from build123d import *

# Parameters (mm, degrees)
SKETCH1_W            = 20
SKETCH1_H            = 6
BOSS_EXTRUDE1_DEPTH  = 21.5
SKETCH2_W            = 6
SKETCH2_H            = 20
BOSS_EXTRUDE2_DEPTH  = 12
SKETCH7_R            = 1.5
CUT_EXTRUDE1_DEPTH   = 46.749316935
SKETCH8_R            = 3.4
CUT_EXTRUDE2_DEPTH   = 30.769951293
FILLET2_R            = 3
CONVERT_SOLID2_START = -10
CONVERT_SOLID2_DEPTH = 20


# Read off the part's stored shape, not the designer's step: Convert-Solid2
with BuildPart() as part:
    # Sketch1 → Boss-Extrude1 (new, symmetric)
    with BuildSketch(Plane(origin=(0, 0, 0), x_dir=(0, 0, -1), z_dir=(1, 0, 0))):
        with Locations((0, -3)):
            Rectangle(SKETCH1_W, SKETCH1_H)
    extrude(amount=BOSS_EXTRUDE1_DEPTH, both=True)

    # Sketch2 → Boss-Extrude2 (add)
    with BuildSketch(Plane(origin=(0, 0, 0), x_dir=(1, 0, 0), z_dir=(0, 1, 0))):
        with Locations((18.5, 0)):
            Rectangle(SKETCH2_W, SKETCH2_H)
        with Locations((-18.5, 0)):
            Rectangle(SKETCH2_W, SKETCH2_H)
    extrude(amount=BOSS_EXTRUDE2_DEPTH)

    # Sketch7 → Cut-Extrude1 (cut, through all)
    with BuildSketch(Plane.ZY.offset(21.5)):
        with Locations((-5, 7)):
            Circle(SKETCH7_R)
        with Locations((5, 7)):
            Circle(SKETCH7_R)
    extrude(amount=-CUT_EXTRUDE1_DEPTH, mode=Mode.SUBTRACT)

    # Sketch8 → Cut-Extrude2 (cut, through all)
    with BuildSketch(Plane.XZ.offset(6)):
        with Locations(Location((0, 0, 0), (0, 0, 270))):
            Circle(SKETCH8_R)
    extrude(amount=-CUT_EXTRUDE2_DEPTH, mode=Mode.SUBTRACT)

    # Fillet2
    fillet2_edges = [part.edges().sort_by_distance(p)[0] for p in [
        (-18.5, 12, 10),
        (-18.5, 12, -10),
        (18.5, 12, -10),
        (18.5, 12, 10),
    ]]
    fillet(fillet2_edges, radius=FILLET2_R)

    # Convert-Solid2 outline → Convert-Solid2 (cut)
    with BuildSketch(Plane.XY.offset(CONVERT_SOLID2_START)):
        with BuildLine():
            Line((21.5, -6), (21.5, 0))
            ThreePointArc((21.5, 0), (19.742640687, -4.242640687), (15.5, -6))
            Line((15.5, -6), (21.5, -6))
        make_face()
        with BuildLine():
            Line((-21.5, -6), (-15.5, -6))
            ThreePointArc((-15.5, -6), (-19.742640687, -4.242640687), (-21.5, 0))
            Line((-21.5, 0), (-21.5, -6))
        make_face()
        with BuildLine():
            Line((19.5, 0), (19.5, 12))
            Line((19.5, 12), (15.5, 12))
            Line((15.5, 12), (15.5, 0))
            Line((15.5, 0), (-15.5, 0))
            Line((-15.5, 0), (-15.5, 12))
            Line((-15.5, 12), (-19.5, 12))
            Line((-19.5, 12), (-19.5, 0))
            ThreePointArc((-19.5, 0), (-18.328427125, -2.828427125), (-15.5, -4))
            Line((-15.5, -4), (15.5, -4))
            ThreePointArc((15.5, -4), (18.328427125, -2.828427125), (19.5, 0))
        make_face()
    extrude(amount=CONVERT_SOLID2_DEPTH, mode=Mode.SUBTRACT)


solid = part.part
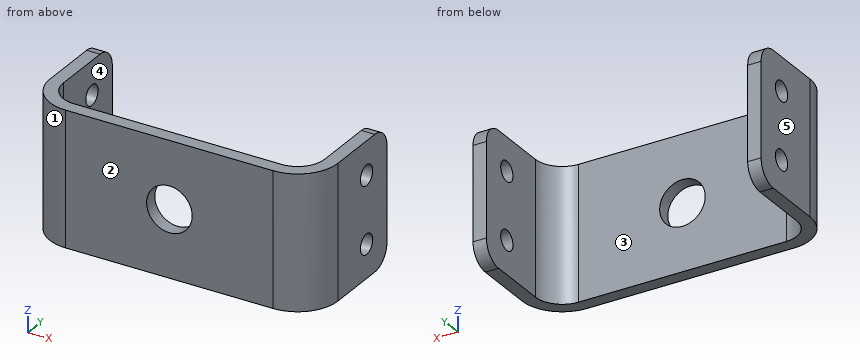
Check sheet for the modelled part. Datum: model origin and axes. Units: mm. Face numbers are marked on the shaded views. A direction names the side the tool comes from. Coordinates: 2 decimals unless noted, no trailing zeros. Loops run counter-clockwise (first coordinate to the right, second up) from the corner with the lowest first, then second, coordinate; pieces in that order, holes last. Notation, with made-up numbers: (42, 82) -> (80, 82) arc R13 cw to (80, 98) -> close; hole circle Ø11 at (-38.75, 70.5). An arc over 180 degrees is marked (long way). Write item = value, one per line. Start each with the question number.
1. Section check C-C on z = 0. Record the cut outline in (x, y).
2. Draft check along X on the marked faces 1, 2 and 3. Enter one of: released by +X, released by -X, zero draft, split by the parting line, or undercut.
3. Section check B-B on z = -5. Record the cut outline in (x, y), then the cut area to 3 significant figures.
4. Depth check by flat-ended pin: P1, Ø10, axis at y = -1, z = -4, coming from the +X side. Enter the tip coordinate at first touch or a pass-through.
5. Tool access check on the marked faces 4 and 5. Record the directions out of +Z, -Z, +X, -X, +Y, -Y that give a thin tool (end or side, any length) a straight path to the whole face; none if there is none.
6. Section check A-A on y = 7. Record the cut outline in (x, z).
7. Material ranges on line 1 (X direction, y = 7, z = -2); line 2 (Y direction, x = 13, z = 1.75); line 3 (X direction, y = -4.6, z = 0), recorded low to high.
8. Section check D-D on y = 4.5. Record the cut outline in (x, z), then the cut area to 3 significant figures.
Responses:
q1.outline = (-21.5, 0) arc R6 ccw to (-15.5, -6) -> (-3.4, -6) -> (-3.4, -4) -> (-15.5, -4) arc R4 cw to (-19.5, 0) -> (-19.5, 12) -> (-21.5, 12) -> close; (3.4, -6) -> (15.5, -6) arc R6 ccw to (21.5, 0) -> (21.5, 12) -> (19.5, 12) -> (19.5, 0) arc R4 cw to (15.5, -4) -> (3.4, -4) -> close
q2.face_1 = released by -X
q2.face_2 = zero draft
q2.face_3 = undercut
q3.outline = (-21.5, 0) arc R6 ccw to (-15.5, -6) -> (15.5, -6) arc R6 ccw to (21.5, 0) -> (21.5, 5.5) -> (19.5, 5.5) -> (19.5, 0) arc R4 cw to (15.5, -4) -> (-15.5, -4) arc R4 cw to (-19.5, 0) -> (-19.5, 5.5) -> (-21.5, 5.5) -> close; (-21.5, 8.5) -> (-19.5, 8.5) -> (-19.5, 12) -> (-21.5, 12) -> close; (19.5, 8.5) -> (21.5, 8.5) -> (21.5, 12) -> (19.5, 12) -> close
q3.area = 129 mm2
q4.P1 = 21.5
q5.face_4 = +Z, -Z, +Y
q5.face_5 = +Z, -Z, -X, +Y, -Y
q6.outline = (-21.5, -10) -> (-19.5, -10) -> (-19.5, -6.5) -> (-21.5, -6.5) -> close; (-21.5, -3.5) -> (-19.5, -3.5) -> (-19.5, 3.5) -> (-21.5, 3.5) -> close; (-21.5, 6.5) -> (-19.5, 6.5) -> (-19.5, 10) -> (-21.5, 10) -> close; (19.5, -10) -> (21.5, -10) -> (21.5, -6.5) -> (19.5, -6.5) -> close; (19.5, -3.5) -> (21.5, -3.5) -> (21.5, 3.5) -> (19.5, 3.5) -> close; (19.5, 6.5) -> (21.5, 6.5) -> (21.5, 10) -> (19.5, 10) -> close
q7.line_1 = -21.5 to -19.5, 19.5 to 21.5
q7.line_2 = -6 to -4
q7.line_3 = -19.35 to -3.4, 3.4 to 19.35
q8.outline = (-21.5, -10) -> (-19.5, -10) -> (-19.5, 10) -> (-21.5, 10) -> close; (19.5, -10) -> (21.5, -10) -> (21.5, 10) -> (19.5, 10) -> close
q8.area = 80.0 mm2
